Design review of the part built by this model. Coordinates are the model's own, in mm. A direction names the side the tool comes from. Round coordinates to 2 decimals unless told otherwise and drop trailing zeros. Order: outer loops, then holes, each group sorted by start corner. A loop starts at its lowest first (then second) coordinate and runs counter-clockwise, first axis right, second up. Notation, with made-up numbers: (-20.5, 50.5) - (16.5, 50.5) arc R23 ccw to (16.5, 71.5) - close; hole circle Ø5 at (37.5, 13). An arc over 180 degrees is marked (long way). Write item = value, one per line.
from build123d import *

# Parameters (mm, degrees)
ESQUISSE1_W             = 27.85
ESQUISSE1_H             = 200
BOSS_EXTRU_2_DEPTH      = 6
ENL_V_MAT_EXTRU_1_DEPTH = 6
ENL_V_START             = -3
ESQUISSE4_R             = 13.925
ENL_V_MAT_EXTRU_2_DEPTH = 3
ESQUISSE5_R             = 3
ENL_V_MAT_EXTRU_3_DEPTH = 3
ESQUISSE6_W             = 17.85
ESQUISSE6_H             = 23
ESQUISSE6_H_2           = 29
ENL_V_MAT_EXTRU_4_DEPTH = 10
CONG_1_R                = 10
CONG_2_R                = 10
ESQUISSE9_W             = 20.2
ESQUISSE9_H             = 40.3
ENL_V_MAT_EXTRU_7_DEPTH = 1.85
ENL_V_MAT_EXTRU_8_DEPTH = 10


with BuildPart() as part:
    # Esquisse1 → Boss.-Extru.2 (new body)
    with BuildSketch(Plane.XY):
        with Locations((1.835077519, -78.788662791)):
            Rectangle(ESQUISSE1_W, ESQUISSE1_H)
        with BuildLine():
            Line((-12.089922481, 21.211337209), (15.760077519, 21.211337209))
            ThreePointArc((15.760077519, 21.211337209), (1.835077519, 35.136337209), (-12.089922481, 21.211337209))
        make_face()
    extrude(amount=BOSS_EXTRU_2_DEPTH)

    # Esquisse3 → Enlèv. mat.-Extru.1 (cut)
    with BuildSketch(Plane.XY.offset(6)):
        with BuildLine():
            Line((4.433153731, -172.288662791), (4.433153731, -169.288662791))
            ThreePointArc((4.433153731, -169.288662791), (-1.164922481, -170.788662791), (4.433153731, -172.288662791))
        make_face()
    extrude(amount=-ENL_V_MAT_EXTRU_1_DEPTH, mode=Mode.SUBTRACT)

    # Esquisse4 → Enlèv. mat.-Extru.2 (cut)
    with BuildSketch(Plane.XY.offset(6).offset(ENL_V_START)):
        with Locations((1.835077519, 21.211337209)):
            Circle(ESQUISSE4_R)
    extrude(amount=ENL_V_MAT_EXTRU_2_DEPTH, mode=Mode.SUBTRACT)

    # Esquisse5 → Enlèv. mat.-Extru.3 (cut)
    with BuildSketch(Plane.XY.offset(3)):
        with Locations((1.835077519, 21.211337209)):
            Circle(ESQUISSE5_R)
    extrude(amount=-ENL_V_MAT_EXTRU_3_DEPTH, mode=Mode.SUBTRACT)

    # Esquisse6 → Enlèv. mat.-Extru.4 (cut)
    with BuildSketch(Plane.XY.offset(6)):
        with BuildLine():
            Line((-7.089922481, -27.788662791), (10.760077519, -27.788662791))
            ThreePointArc((10.760077519, -27.788662791), (1.835077519, -18.863662791), (-7.089922481, -27.788662791))
        make_face()
        with Locations((1.835077519, -39.288662791)):
            Rectangle(ESQUISSE6_W, ESQUISSE6_H)
        with BuildLine():
            Line((-7.089922481, -50.788662791), (10.760077519, -50.788662791))
            ThreePointArc((10.760077519, -50.788662791), (1.835077519, -59.713662791), (-7.089922481, -50.788662791))
        make_face()
        with BuildLine():
            ThreePointArc((-7.089922481, -73.788662791), (1.835077519, -64.863662791), (10.760077519, -73.788662791))
            Line((10.760077519, -73.788662791), (-7.089922481, -73.788662791))
        make_face()
        with Locations((1.835077519, -88.288662791)):
            Rectangle(ESQUISSE6_W, ESQUISSE6_H_2)
        with BuildLine():
            Line((-7.089922481, -102.788662791), (10.760077519, -102.788662791))
            ThreePointArc((10.760077519, -102.788662791), (1.835077519, -111.713662791), (-7.089922481, -102.788662791))
        make_face()
        with BuildLine():
            Line((-7.089922481, -125.788662791), (10.760077519, -125.788662791))
            ThreePointArc((10.760077519, -125.788662791), (1.835077519, -116.863662791), (-7.089922481, -125.788662791))
        make_face()
        with Locations((1.835077519, -137.288662791)):
            Rectangle(ESQUISSE6_W, ESQUISSE6_H)
        with BuildLine():
            Line((-7.089922481, -148.788662791), (10.760077519, -148.788662791))
            ThreePointArc((10.760077519, -148.788662791), (1.835077519, -157.713662791), (-7.089922481, -148.788662791))
        make_face()
    extrude(amount=-ENL_V_MAT_EXTRU_4_DEPTH, mode=Mode.SUBTRACT)

    # Congé1
    cong_1_edges = [part.edges().sort_by_distance(p)[0] for p in [
        (-12.089922481, -178.788662791, 3),
    ]]
    fillet(cong_1_edges, radius=CONG_1_R)

    # Congé2
    cong_2_edges = [part.edges().sort_by_distance(p)[0] for p in [
        (15.760077519, -178.788662791, 3),
    ]]
    fillet(cong_2_edges, radius=CONG_2_R)

    # Esquisse9 → Enlèv. mat.-Extru.7 (cut)
    with BuildSketch(Plane(origin=(0, 0, 0), x_dir=(-1, 0, 0), z_dir=(0, 0, -1))):
        with Locations((-1.830077519, 10.911337209)):
            Rectangle(ESQUISSE9_W, ESQUISSE9_H)
    extrude(amount=-ENL_V_MAT_EXTRU_7_DEPTH, mode=Mode.SUBTRACT)

    # Esquisse11 → Enlèv. mat.-Extru.8 (cut)
    # profile 1 of 7: a face of its own
    with BuildSketch(Plane.XY.offset(6)):
        Polygon((-2.060393609, -172.284133919), (-2.060393609, -169.293191663), (-3.673950582, -170.788662791), align=None)
    # profile 2 of 7: a face of its own
    with BuildSketch(Plane.XY.offset(6)):
        Polygon((0.339606391, -166.893191663), (-2.060393609, -166.893191663), (-2.060393609, -169.293191663), (-2.060393609, -172.284133919), (-2.060393609, -174.684133919), (0.339606391, -174.684133919), (3.330548647, -174.684133919), (5.730548647, -174.684133919), (5.730548647, -172.284133919), (5.730548647, -169.293191663), (5.730548647, -166.893191663), (3.330548647, -166.893191663), align=None)
        with BuildLine():
            ThreePointArc((4.433153731, -172.288662791), (-1.164922481, -170.788662791), (4.433153731, -169.288662791))
            ThreePointArc((4.433153731, -169.288662791), (4.732854998, -170.012205655), (4.835077519, -170.788662791))
            ThreePointArc((4.835077519, -170.788662791), (4.732854998, -171.565119926), (4.433153731, -172.288662791))
        make_face(mode=Mode.SUBTRACT)
    # profile 3 of 7: a face of its own
    with BuildSketch(Plane.XY.offset(6)):
        Polygon((1.835077519, -165.27963469), (0.339606391, -166.893191663), (3.330548647, -166.893191663), align=None)
    # profile 4 of 7: a face of its own
    with BuildSketch(Plane.XY.offset(6)):
        Polygon((7.34410562, -170.788662791), (5.730548647, -169.293191663), (5.730548647, -172.284133919), align=None)
    # profile 5 of 7: a face of its own
    with BuildSketch(Plane.XY.offset(6)):
        Polygon((3.330548647, -174.684133919), (0.339606391, -174.684133919), (1.835077519, -176.297690892), align=None)
    # profile 6 of 7: a face of its own
    with BuildSketch(Plane.XY.offset(6)):
        with BuildLine():
            ThreePointArc((4.835077519, -170.788662791), (4.732854998, -170.012205655), (4.433153731, -169.288662791))
            Line((4.433153731, -169.288662791), (4.433153731, -172.288662791))
            ThreePointArc((4.433153731, -172.288662791), (4.732854998, -171.565119926), (4.835077519, -170.788662791))
        make_face()
    # profile 7 of 7: a face of its own
    with BuildSketch(Plane.XY.offset(6)):
        with BuildLine():
            Line((4.433153731, -172.288662791), (4.433153731, -169.288662791))
            ThreePointArc((4.433153731, -169.288662791), (-1.164922481, -170.788662791), (4.433153731, -172.288662791))
        make_face()
    extrude(amount=-ENL_V_MAT_EXTRU_8_DEPTH, mode=Mode.SUBTRACT)


solid = part.part
1) The part is to be moulded in two halves that separate along X. For faces 5 (the flat face through (10.76, -137, 3)), 6 (the cylindrical face through (-9.24, -175.78, 3.04)), 7 (the flat face through (2, 33, 0)), say which applies: released by +X, released by -X, zero draft, split by the parting line, or undercut.
Findings:
face_5 = undercut
face_6 = released by -X
face_7 = zero draft
2) We need section C-C on y = 13. Write out the cut boundary in (x, z).
Findings:
outline = (-12.09, 0) - (-8.27, 0) - (-8.27, 1.85) - (11.93, 1.85) - (11.93, 0) - (15.76, 0) - (15.76, 6) - (13.08, 6) - (13.08, 3) - (-9.41, 3) - (-9.41, 6) - (-12.09, 6) - close
3) To check wall thickness, follow L1, parallel to X at y = -135, z = 2.75; L2, parallel to Y at x = 3.25, z = 2.5; L3, parallel to Y at x = 6.25, z = 2.5. State the ranges of each line that lie inside material, in increasing order. Write a range as from..to.
Findings:
L1 = -12.09..-7.09, 10.76..15.76
L2 = -178.79..-174.77, -166.81..-157.6, -116.98..-111.6, -64.98..-59.6, -18.98..18.57, 23.86..35.06
L3 = -178.78..-171.8, -169.77..-156.55, -118.03..-110.55, -66.03..-58.55, -20.03..34.42
4) Clearance check with flat-ended pins moving along their axes: pin 1 Ø5 at (x, y) = (-8, 4) entering from -Z; pin 2 Ø1.2 at (y, z) = (-174, 3) entering from +X; pin 3 Ø0.9 at (x, z) = (-3, 0.5) entering from +Y; pin 4 Ø1.9 at (x, z) = (-1, 2.5) entering from +Y. State where each tip first meets the part, or that it passes through.
Findings:
pin_1 = 0
pin_2 = 14.63
pin_3 = 34.43
pin_4 = 35.01
5) We need section B-B on y = -109. Write out the cut boundary in (x, z).
Findings:
outline = (-12.09, 0) - (-4.57, 0) - (-4.57, 6) - (-12.09, 6) - close; (8.24, 0) - (15.76, 0) - (15.76, 6) - (8.24, 6) - close
6) We need section A-A on y = -79.5. Write out the cut boundary in (x, z), and give its area (3 significant figures).
Findings:
outline = (-12.09, 0) - (-7.09, 0) - (-7.09, 6) - (-12.09, 6) - close; (10.76, 0) - (15.76, 0) - (15.76, 6) - (10.76, 6) - close
area = 60.0 mm^2
7) For faces 1 (the cylindrical face through (1.53, 7.29, 4.48)), 2 (the cylindrical face through (12.75, -175.94, 3.04)), 3 (the cylindrical face through (1.639, -64.866, 3.042)), 4 (the flat face through (2, 11, 1.85)), list the 3-axis set-ups (+Z, -Z, +X, -X, +Y, -Y) from which the entire face can be reached by the end or side of a thin tool; tool diameter is ignored.
Findings:
face_1 = +Z, +Y
face_2 = +Z, -Z, +X, -Y
face_3 = +Z, -Z
face_4 = -Z
